```python
from build123d import *

# Parameters (mm, degrees)
EXTRUDE_1_DEPTH     = 5
CUT_EXTRUDE_1_DEPTH = 10


with BuildPart() as part:
    # 草图1 → 凸台-拉伸1 (new body)
    with BuildSketch(Plane.XY):
        with BuildLine():
            Line((-59, -25), (-59, -32))
            ThreePointArc((-59, -32), (-58.121320344, -34.121320344), (-56, -35))
            Line((-56, -35), (56, -35))
            ThreePointArc((56, -35), (58.121320344, -34.121320344), (59, -32))
            Line((59, -32), (59, -25))
            Line((59, -25), (59, 25))
            ThreePointArc((59, 25), (58.121320344, 27.121320344), (56, 28))
            Line((56, 28), (-56, 28))
            ThreePointArc((-56, 28), (-58.121320344, 27.121320344), (-59, 25))
            Line((-59, 25), (-59, -25))
        make_face()
        with BuildLine():
            Line((12.85, -17), (12.85, 17))
            ThreePointArc((12.85, 17), (15, 19.15), (17.15, 17))
            Line((17.15, 17), (17.15, -17))
            ThreePointArc((17.15, -17), (15, -19.15), (12.85, -17))
        make_face(mode=Mode.SUBTRACT)
        with BuildLine():
            Line((-12.85, -17), (-12.85, 17))
            ThreePointArc((-12.85, 17), (-15, 19.15), (-17.15, 17))
            Line((-17.15, 17), (-17.15, -17))
            ThreePointArc((-17.15, -17), (-15, -19.15), (-12.85, -17))
        make_face(mode=Mode.SUBTRACT)
    extrude(amount=EXTRUDE_1_DEPTH)

    # 草图2 → 切除-拉伸1 (cut)
    with BuildSketch(Plane.XY.offset(5)):
        with BuildLine():
            Line((-47.75, 16.25), (-42.5, 16.25))
            ThreePointArc((-42.5, 16.25), (-39.25, 13), (-42.5, 9.75))
            Line((-42.5, 9.75), (-47.75, 9.75))
            ThreePointArc((-47.75, 9.75), (-51, 13), (-47.75, 16.25))
        make_face()
        with BuildLine():
            Line((-47.75, -23.25), (-42.5, -23.25))
            ThreePointArc((-42.5, -23.25), (-39.25, -20), (-42.5, -16.75))
            Line((-42.5, -16.75), (-47.75, -16.75))
            ThreePointArc((-47.75, -16.75), (-51, -20), (-47.75, -23.25))
        make_face()
        with BuildLine():
            Line((47.75, 16.25), (42.5, 16.25))
            ThreePointArc((42.5, 16.25), (39.25, 13), (42.5, 9.75))
            Line((42.5, 9.75), (47.75, 9.75))
            ThreePointArc((47.75, 9.75), (51, 13), (47.75, 16.25))
        make_face()
        with BuildLine():
            Line((47.75, -23.25), (42.5, -23.25))
            ThreePointArc((42.5, -23.25), (39.25, -20), (42.5, -16.75))
            Line((42.5, -16.75), (47.75, -16.75))
            ThreePointArc((47.75, -16.75), (51, -20), (47.75, -23.25))
        make_face()
    extrude(amount=-CUT_EXTRUDE_1_DEPTH, mode=Mode.SUBTRACT)


solid = part.part
```
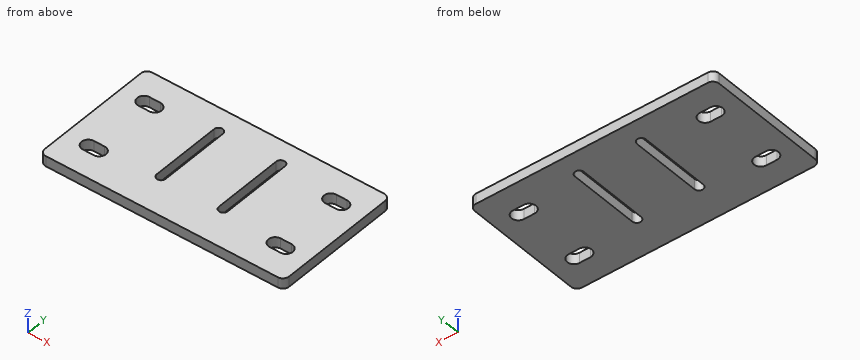
Could you check a few things on this model? Use its own coordinates, in mm. Coordinates: 2 decimals unless noted, no trailing zeros. Write each loop counter-clockwise with the first axis right and the second up, starting at its lowest first coordinate (ties: lowest second). Pieces come first, ordered by that corner, then holes. Notation, with made-up numbers: (-7, -0.5) -> (43, -0.5) arc R10 ccw to (43, 9.5) -> close; hole circle Ø1 at (-14, 22). An arc over 180 degrees is marked (long way). Write item = value, one per line. Start each with the question number.
(1) I want a section at A-A (y = 1.5). Please give me the cut outline in (x, z), plus the area to 3 significant figures.
(2) I want a section at D-D (y = 13). Please give me the cut outline in (x, z).
(3) I want a section at C-C (z = 2.55). Give the number of separate pieces and of enclosed holes in the cut face, plus the area to 3 significant figures.
(4) I need wall thicknesses on line 1 (X direction, y = -16.5, z = 2.75); line 2 (Y direction, x = 44.5, z = 1.45); line 3 (Y direction, x = -39.5, z = 0.6). Which ranges of each line are inside material? Lowest first, please. Write a range as [from, to].
(5) I want a section at B-B (x = -15). Please give me the cut outline in (y, z).
(6) Will this pin go through, and if not, where does the flat tip stop? pin 1 (3 mm diameter, centred on x = -18.5, y = 7, fed in from -Z).
Result set:
q1.outline = (-59, 0) -> (-17.15, 0) -> (-17.15, 5) -> (-59, 5) -> close; (-12.85, 0) -> (12.85, 0) -> (12.85, 5) -> (-12.85, 5) -> close; (17.15, 0) -> (59, 0) -> (59, 5) -> (17.15, 5) -> close
q1.area = 547 mm2
q2.outline = (-59, 0) -> (-51, 0) -> (-51, 5) -> (-59, 5) -> close; (-39.25, 0) -> (-17.15, 0) -> (-17.15, 5) -> (-39.25, 5) -> close; (-12.85, 0) -> (12.85, 0) -> (12.85, 5) -> (-12.85, 5) -> close; (17.15, 0) -> (39.25, 0) -> (39.25, 5) -> (17.15, 5) -> close; (51, 0) -> (59, 0) -> (59, 5) -> (51, 5) -> close
q3.separate_pieces = 1
q3.enclosed_holes = 6
q3.area = 6,840 mm2
q4.line_1 = [-59, -17.15], [-12.85, 12.85], [17.15, 59]
q4.line_2 = [-35, -23.25], [-16.75, 9.75], [16.25, 28]
q4.line_3 = [-35, -21.25], [-18.75, 11.75], [14.25, 28]
q5.outline = (-35, 0) -> (-19.15, 0) -> (-19.15, 5) -> (-35, 5) -> close; (19.15, 0) -> (28, 0) -> (28, 5) -> (19.15, 5) -> close
q6.pin_1 = 0
